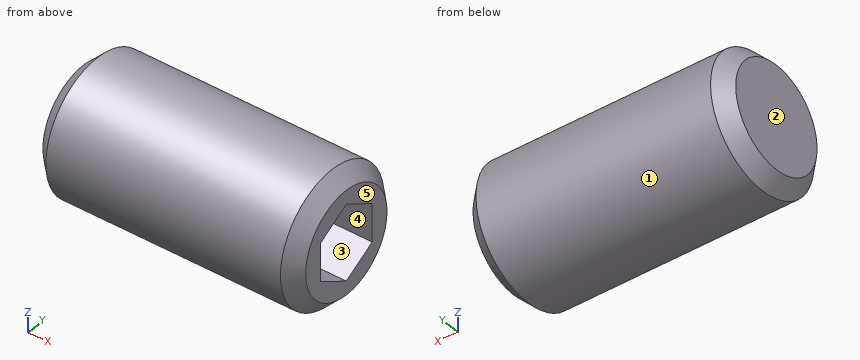
Autodesk Inventor part; units mm, degrees
ref_plane "Work Plane1" through (4, 0, 0) normal (0, 0.5, 0.866) x (1, 0, 0)
ref_plane "YZ Plane" through (0, 0, 0) normal (1, 0, 0) x (0, 1, 0)
ref_plane "XZ Plane" through (0, 0, 0) normal (0, 1, 0) x (-1, 0, 0)
sketch "Sketch1" plane through (0, 0, 0) normal (0, 0, 1) x (1, 0, 0)
  line L0 (0, 0) -> (4.8333, 0)
  line L1 (8, 1.1547) -> (8, 2)
  line L2 (8, 2) -> (0, 2)
  line L3 (8, 1.1547) -> (5.5, 1.1547)
  line L4 (5.5, 1.1547) -> (4.8333, 0)
  line L5 (0, -0.4) -> (0, 2.4)
  line L6 (0, 2) -> (0, 0)
  dimension "d0" = 2.5
  dimension "d1" = 60
  dimension "d2" = 4
  dimension "d3" = 2.3094
  dimension "d5" = 8
revolve "Body" add sketch "Sketch1" angle 360 about axis through (0, 0, 0) along (1, 0, 0)
chamfer "Chamfer1" distance 0.4294 angle 45 1 edges at (8, -2, 0) measured on face at (8, 1.6877, -0.2517)
sketch "Sketch2" plane through (8, 0, 0) normal (1, 0, 0) x (0, 0, -1)
  circle A0 centre (0, 0) radius 1.1547
  line L0 (-0.5774, 1) -> (0.5774, 1)
  line L1 (0.5774, 1) -> (1.1547, 0)
  line L2 (1.1547, 0) -> (0.5774, -1)
  line L3 (0.5774, -1) -> (-0.5774, -1)
  line L4 (-0.5774, -1) -> (-1.1547, 0)
  line L5 (-1.1547, 0) -> (-0.5774, 1)
extrude "Slot" add sketch "Sketch2" against normal up to next contours L1 A0 | A0 L2 | L0 A0 | A0 L3 | L5 A0 | A0 L4
thread "Thread"
chamfer "Chamfer2" distance 0.4294 angle 45 1 edges at (0, -2, 0) measured on face at (2.5235, 1.9935, -0.1609)
ref_plane "Work Plane1" through (4, 0, 0) normal (0, 0.5, 0.866) x (1, 0, 0)
equation "\"d0\" = INTI"
equation "\"d2\" = NND"
equation "\"d3\" = 1.1547 * SW"
equation "\"d5\" = NLG"
equation "\"d7\" = -0.5 * GD1 + 0.5 * NND"
equation "\"d8\" = FAWI"
equation "\"d29\" = -0.5 * GD1 + 0.5 * NND"
equation "\"d11\" = NLG"
equation "\"d13\" = -0.5 * GD1 + 0.5 * NND"
equation "\"d14\" = FAWI"
equation "\"d30\" = -0.5 * GD1 + 0.5 * NND"
equation "\"NND\" = 4"
equation "\"NLG\" = 8"
equation "\"INTI\" = 2.5"
equation "\"FAWI\" = 45deg"
equation "\"SW\" = 2"
equation "\"GD1\" = THREADDIA - 1.2269 * PTC"
equation "\"FAWI1\" = 45deg"
equation "\"GUL\" = 0.61345 * PTC"
equation "\"SPD\" = 2.5"
equation "\"SEWI\" = 90deg"
equation "\"TOA\" = 30deg"
equation "\"THREADDIA\" = 4"
equation "\"PTC\" = 0.7"
equation "\"GAL\" = 0.61345 * PTC"
equation "\"E0\" = 1.155 * SW"
properties part number "ISO 4026 - M4 x 8(1)" material "Stainless Steel, 440C"
Read the model definition and answer for the solid it produces. Units are mm, in the model's axes. Face numbers are marked on the shaded views. A direction names the side the tool comes from. Round coordinates to 2 decimals unless told otherwise and drop trailing zeros. Write each loop counter-clockwise with the first axis right and the second up, starting at its lowest first coordinate (ties: lowest second). Pieces come first, ordered by that corner, then holes.
1. Which of the six approach directions +Z, -Z, +X, -X, +Y, -Y give full straight-line access (tool end or side, diameter ignored) to the marked faces 4 and 5?
2. Straight lines are drawn through the part: L1, parallel to Z at x = 7.75, y = -0.25; L2, parallel to Z at x = 2, y = 1.8; L3, parallel to Z at x = 0.75, y = 0.4. For each, find the intervals that lie inside material, in ascending order.
3. The part is cut by section A-A, the plane x = 3.5. Determine the outline of the cut face in (y, z).
4. Determine the mould class of the marked faces 1, 2 and 3 for opening direction Z: pulls with the +Z half, pulls with the -Z half, needs draft (parallel to the pull), parting line crosses it, or undercut.
5. Given pin 1 Ø2 at (y, z) = (-0.5, 0) entering from -X, flat-ended and moving along its own axis, determine where the tip first touches the part or whether it passes through.
Values:
1. face 4: +X
1. face 5: +Z, -Z, +X, +Y, -Y
2. L1: z = -1.8 to -1.01, 1.01 to 1.8
2. L2: z = -0.87 to 0.87
2. L3: z = -1.96 to 1.96
3. outline: circle Ø4 at (0, 0)
4. face 1: parting line crosses it
4. face 2: needs draft
4. face 3: undercut
5. pin 1: stops at x = 0
